For this review, use the dimensioned drawing (mm, ordinates from the lowest corner) and the shaded views. Round coordinates to 2 decimals unless told otherwise and drop trailing zeros. Order: outer loops, then holes, each group sorted by start corner. A loop starts at its lowest first (then second) coordinate and runs counter-clockwise, first axis right, second up. Notation, with made-up numbers: M -26.75,80.25 L 21.25,80.25 A9 ccw 21.25,85.25 Z; hole C 45,76.5 d2. An arc over 180 degrees is marked long. Put each result on its own line as item: value.
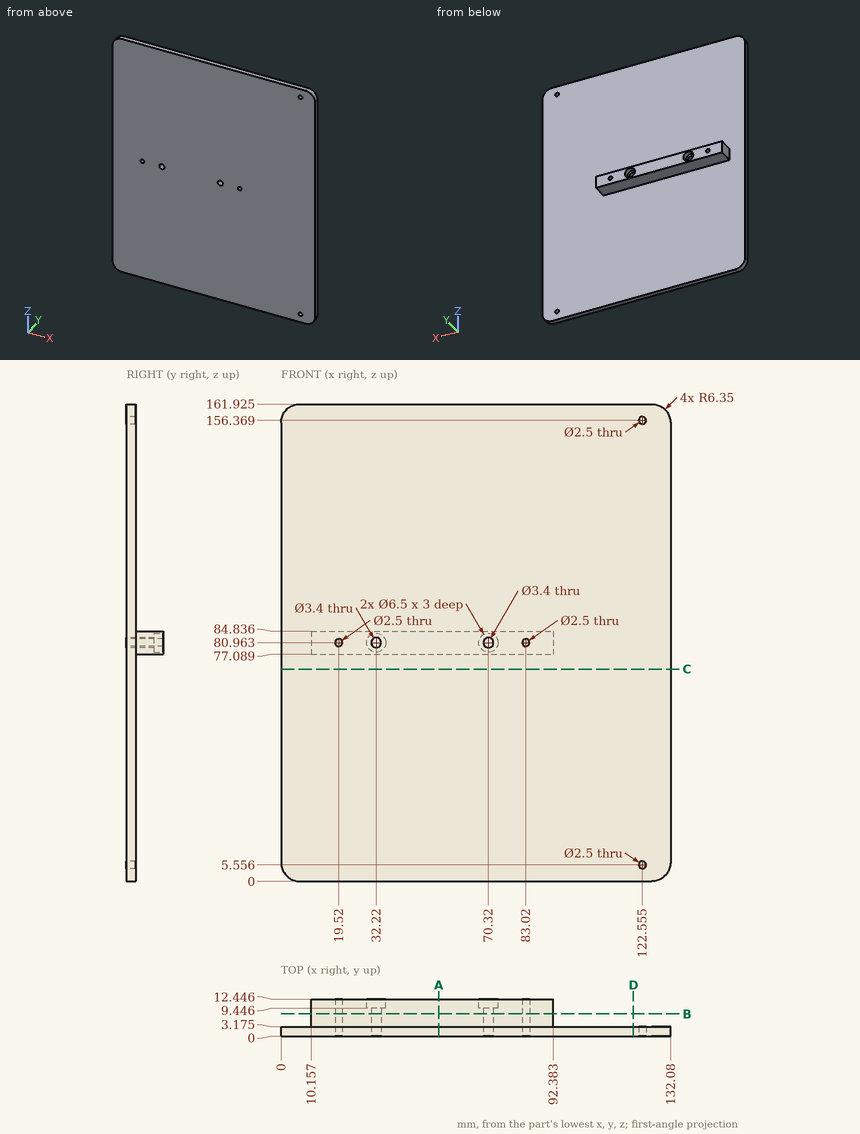
(1) Add section B-B on y = 7.5. State how many separate pieces and enclosed holes the cut face has, then the cut area to 3 significant figures.
A:
separate pieces: 1
enclosed holes: 4
area: 609 mm2
(2) Add section C-C on z = 72. Give the boundary of the cut face in (x, y) (1 decimal).
A:
outline: M 0,0 L 132.1,0 L 132.1,3.2 L 0,3.2 Z
(3) Add section D-D on x = 119.5. Give the boundary of the cut face in (y, z) (1 decimal), then the cut area to 3 significant figures.
A:
outline: M 0,0 L 3.2,0 L 3.2,161.9 L 0,161.9 Z
area: 514 mm2
(4) Add section A-A on x = 53.5. Give the boundary of the cut face in (y, z) (1 decimal), then the cut area to 3 significant figures.
A:
outline: M 0,0 L 3.2,0 L 3.2,77.1 L 12.4,77.1 L 12.4,84.8 L 3.2,84.8 L 3.2,161.9 L 0,161.9 Z
area: 586 mm2
(5) To check wall thickness, follow L1, parallel to Y at x = 65, z = 147.5 (1 decimal); L2, parallel to Z at x = 59, y = 9.5 (1 decimal); L3, parallel to Z at x = 69, y = 9.5 (1 decimal). State the ranges of each line that lie inside material, in increasing order.
A:
L1: y = 0 to 3.2
L2: z = 77.1 to 84.8
L3: z = 77.1 to 78, 83.9 to 84.8
(6) Insertion check: pin 1 Ø2.5 at (y, z) = (10, 82.5) entering from -X; pin 2 Ø4 at (x, z) = (70.32, 80.96) entering from -Y; pin 3 Ø1 at (x, y) = (39, 9.5) entering from -Z; pin 4 Ø3 at (x, z) = (70.32, 80.96) entering from -Y. Each pin has a flat end and moves straight along its axis. Give the tip position at first contact, or say it passes through.
A:
pin 1: stops at x = 10.16
pin 2: stops at y = 0
pin 3: stops at z = 77.09
pin 4: passes through
